Model file for the job. Use its own axes, mm. A direction names the side the tool comes from. Coordinates: 2 decimals unless noted, no trailing zeros. Write each loop counter-clockwise with the first axis right and the second up, starting at its lowest first coordinate (ties: lowest second). Pieces come first, ordered by that corner, then holes. Notation, with made-up numbers: (86.25, -7.5) -> (137.25, -7.5) arc R4 ccw to (137.25, -0.5) -> close; hole circle Ø8 at (83, 87.25). An arc over 180 degrees is marked (long way). Write item = value, one per line. Start each with the question number.
from build123d import *

# Parameters (mm, degrees)
BOSS_EXTRUDE1_DEPTH = 150
FILLET1_R           = 10
CUT_EXTRUDE1_DEPTH  = 200.060292374
FILLET2_R           = 10
SKETCH3_W           = 90
SKETCH3_H           = 145
CUT_EXTRUDE2_DEPTH  = 55
FILLET3_R           = 5


with BuildPart() as part:
    # Sketch1 → Boss-Extrude1 (new body)
    with BuildSketch(Plane.XY):
        Polygon((-47.5, 90), (-47.5, 0), (-42.5, 0), (-42.5, 30), (42.5, 30), (42.5, 0), (47.5, 0), (47.5, 90), align=None)
    extrude(amount=-BOSS_EXTRUDE1_DEPTH)

    # Fillet1
    fillet1_edges = [part.edges().sort_by_distance(p)[0] for p in [
        (-45, 0, 0),
        (45, 0, -150),
        (45, 0, 0),
        (-45, 0, -150),
    ]]
    fillet(fillet1_edges, radius=FILLET1_R)

    # Sketch2 → Cut-Extrude1 (cut, through all)
    with BuildSketch(Plane(origin=(47.5, 0, 0), x_dir=(0, 0, -1), z_dir=(1, 0, 0))):
        with BuildLine():
            Line((140, 20), (140, 30))
            Line((140, 30), (10, 30))
            Line((10, 30), (10, 20))
            ThreePointArc((10, 20), (12.928932188, 12.928932188), (20, 10))
            Line((20, 10), (130, 10))
            ThreePointArc((130, 10), (137.071067812, 12.928932188), (140, 20))
        make_face()
    extrude(amount=-CUT_EXTRUDE1_DEPTH, mode=Mode.SUBTRACT)

    # Fillet2
    fillet2_edges = [part.edges().sort_by_distance(p)[0] for p in [
        (-45, 30, -140),
        (-45, 30, -10),
        (45, 30, -140),
        (45, 30, -10),
    ]]
    fillet(fillet2_edges, radius=FILLET2_R - 0.0001)  # a hair under: the kernel refuses the full size

    # Sketch3 → Cut-Extrude2 (cut)
    with BuildSketch(Plane(origin=(0, 90, 0), x_dir=(1, 0, 0), z_dir=(0, 1, 0))):
        with Locations((0, 75)):
            Rectangle(SKETCH3_W, SKETCH3_H)
    extrude(amount=-CUT_EXTRUDE2_DEPTH, mode=Mode.SUBTRACT)

    # Fillet3
    fillet3_edges = [part.edges().sort_by_distance(p)[0] for p in [
        (42.5, 30, -140.00005),
        (-42.5, 30, -140.00005),
        (-42.5, 30, -9.99995),
        (42.5, 30, -9.99995),
    ]]
    fillet(fillet3_edges, radius=FILLET3_R)


solid = part.part
(1) 3-axis set-ups, long thin cutter, end or side, ignore diameter. For faces 1 (the face through (-45, 63, -74)), 2 (the face through (-47.5, 56, -74)), 3 (the face through (41, 28.57, -7.64)), 4 (the face through (-44.96, 12.85, -136.99)): which of +Z, -Z, +X, -X, +Y, -Y reach the whole face in a straight line?
(2) Drill centre lines: line 1 along X through (y, z) = (57, -23.5); line 2 along Z through (x, y) = (17.5, 69); line 3 along X through (y, z) = (9.5, -71). Where is each one in solid material? Low to high.
(3) Saw through at C-C (x = -17.5). Give the cut face in (y, z), then the cut area to 4 significant figures.
(4) Saw through at B-B (y = 82). Give the cut face in (x, z), then the cut area to 3 significant figures.
(5) Drop flat-ended pins along their axis: pin 1 Ø4 at (x, z) = (4.5, -93) entering from +Y; pin 2 Ø5 at (y, z) = (14, -50.5) entering from +X; pin 3 Ø1.5 at (x, z) = (-13, -114) entering from -Y. Give the stop position or say it passes through.
(6) Mould opens along Z. For faces 5 (the face through (1, 30, -76)), 6 (the face through (45, 0, -74)), 7 (the face through (-1, 59, 0)) say: released by +Z, released by -Z, zero draft, split by the parting line, or undercut.
(7) Saw through at A-A (z = -42). Give the cut face in (x, y).
(8) Saw through at D-D (y = 28). Give the cut face in (x, z), then the cut area to 3 significant figures.
Returned:
q1.face_1 = +Y
q1.face_2 = +Z, -Z, -X, +Y, -Y
q1.face_3 = +Z, -Z, -Y
q1.face_4 = +X, -X
q2.line_1 = -47.5 to -45, 45 to 47.5
q2.line_2 = -150 to -147.5, -2.5 to 0
q2.line_3 = -47.5 to -42.5, 42.5 to 47.5
q3.outline = (30, -150) -> (90, -150) -> (90, -147.5) -> (35, -147.5) -> (35, -2.5) -> (90, -2.5) -> (90, 0) -> (30, 0) -> close
q3.area = 1,025 mm2
q4.outline = (-47.5, -150) -> (47.5, -150) -> (47.5, 0) -> (-47.5, 0) -> close; hole (-45, -147.5) -> (45, -147.5) -> (45, -2.5) -> (-45, -2.5) -> close
q4.area = 1,200 mm2
q5.pin_1 = 35
q5.pin_2 = through
q5.pin_3 = 30
q6.face_5 = undercut
q6.face_6 = zero draft
q6.face_7 = released by +Z
q7.outline = (-47.5, 0) -> (-42.5, 0) -> (-42.5, 10) -> (-47.5, 10) -> close; (-47.5, 30) -> (47.5, 30) -> (47.5, 90) -> (45, 90) -> (45, 35) -> (-45, 35) -> (-45, 90) -> (-47.5, 90) -> close; (42.5, 0) -> (47.5, 0) -> (47.5, 10) -> (42.5, 10) -> close
q8.outline = (-47.5, -150) -> (-41.5, -150) -> (-41.5, -136) -> (-47.5, -136) -> close; (-47.5, -14) -> (-41.5, -14) -> (-41.5, 0) -> (-47.5, 0) -> close; (41.5, -150) -> (47.5, -150) -> (47.5, -136) -> (41.5, -136) -> close; (41.5, -14) -> (47.5, -14) -> (47.5, 0) -> (41.5, 0) -> close
q8.area = 336 mm2
